Source: CAD feature listing. Evaluate the final solid. Frame: model axes, mm. Give positions to 0.01 mm unless a question says otherwise; leave off trailing zeros. Loops run counter-clockwise (first coordinate to the right, second up) from the corner with the lowest first, then second, coordinate; pieces in that order, holes last. Notation, with made-up numbers: (78.5, 78) - (119.5, 78) arc R13 cw to (119.5, 93) - close; hole circle Ø10 at (33.5, 77). An arc over 180 degrees is marked (long way). Put each result on its own line as item: value.
Autodesk Inventor part; units mm, degrees
ref_plane "YZ Plane" through (0, 0, 0) normal (1, 0, 0) x (0, 1, 0)
ref_plane "XZ Plane" through (0, 0, 0) normal (0, 1, 0) x (-1, 0, 0)
ref_plane "XY Plane" through (0, 0, 0) normal (0, 0, 1) x (1, 0, 0)
sketch "草图1" plane through (0, 0, 0) normal (1, 0, 0) x (0, 1, 0)
  circle A0 centre (0, 0) radius 65
  circle A1 centre (0, 0) radius 41
  circle A2 centre (52.5, 0) radius 5.5
  circle A3 centre (0, 52.5) radius 5.5
  circle A4 centre (-52.5, 0) radius 5.5
  circle A5 centre (0, -52.5) radius 5.5
  dimension "d1" = 130
  dimension "d3" = 82
  dimension "d4" = 11
  dimension "d5" = 52.5
  dimension "d8" = 360
extrude "拉伸1" add sketch "草图1" along normal blind 0.5
equation "\"d1\" = D2"
equation "\"d3\" = d2"
equation "\"d4\" = d0"
equation "\"d10\" = b"
equation "\"b\" = 0.5"
equation "\"d0\" = 11"
equation "\"D0\" = 105"
equation "\"d2\" = 82"
equation "\"D2\" = 130"
properties part number "低速轴承调整垫片" material "铜，锻铸"
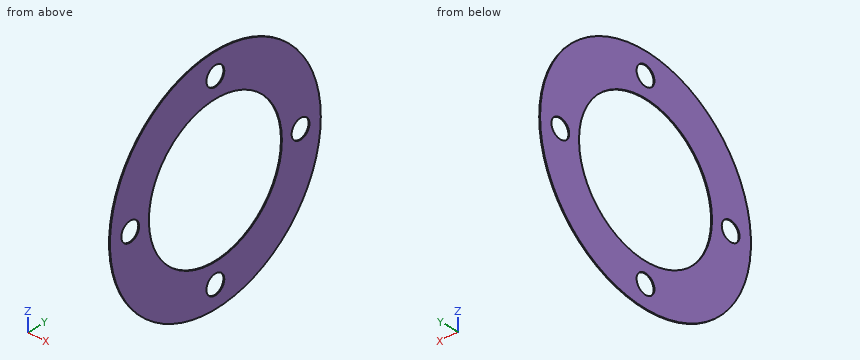
1) Material intervals for line 1 along Z through (x, y) = (0.2, 0); line 2 along Z through (x, y) = (0.2, -4.5); line 3 along Z through (x, y) = (0.2, -52.5), sorted ascending. Write a range as [from, to].
Check result:
line 1: [-65, -58], [-47, -41], [41, 47], [58, 65]
line 2: [-64.84, -55.66], [-49.34, -40.75], [40.75, 49.34], [55.66, 64.84]
line 3: [-38.32, -5.5], [5.5, 38.32]
2) Section query C-C, the plane z = -52.5. Output: boundary loops of the cut face in (x, y).
Check result:
outline: (0, -38.32) - (0.5, -38.32) - (0.5, -5.5) - (0, -5.5) - close; (0, 5.5) - (0.5, 5.5) - (0.5, 38.32) - (0, 38.32) - close
3) Section query A-A, the plane x = 0.35. Output: boundary loops of the cut face in (y, z), plus the area to 3 significant figures.
Check result:
outline: circle Ø130 at (0, 0); hole circle Ø11 at (-52.5, 0); hole circle Ø82 at (0, 0); hole circle Ø11 at (0, -52.5); hole circle Ø11 at (0, 52.5); hole circle Ø11 at (52.5, 0)
area: 7,610 mm²
4) Section query B-B, the plane y = 10.5. Output: boundary loops of the cut face in (x, z).
Check result:
outline: (0, -64.15) - (0.5, -64.15) - (0.5, -39.63) - (0, -39.63) - close; (0, 39.63) - (0.5, 39.63) - (0.5, 64.15) - (0, 64.15) - close
5) Section query D-D, the plane z = 2.5. Output: boundary loops of the cut face in (x, y).
Check result:
outline: (0, -64.95) - (0.5, -64.95) - (0.5, -57.4) - (0, -57.4) - close; (0, -47.6) - (0.5, -47.6) - (0.5, -40.92) - (0, -40.92) - close; (0, 40.92) - (0.5, 40.92) - (0.5, 47.6) - (0, 47.6) - close; (0, 57.4) - (0.5, 57.4) - (0.5, 64.95) - (0, 64.95) - close
